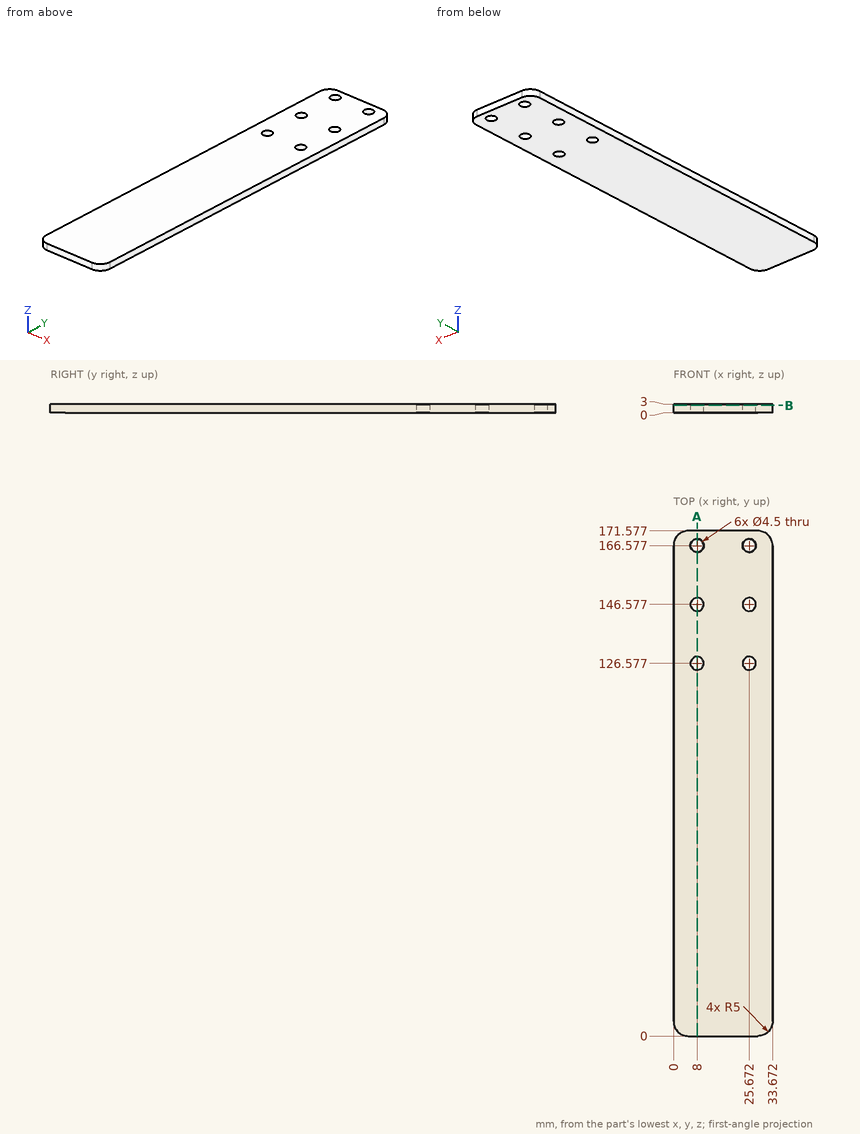
Check sheet for the drawn part. Datum: minimum x, y, z corner. Units: mm. Round coordinates to 2 decimals unless told otherwise and drop trailing zeros. Loops run counter-clockwise (first coordinate to the right, second up) from the corner with the lowest first, then second, coordinate; pieces in that order, holes last.
Item 1: Cross-section at A-A on x = 8. Record the boundary of the cut face in (y, z).
Item 2: Cross-section at B-B on z = 2.5. Record the boundary of the cut face in (x, y), then the cut area to 3 significant figures.
Item 3: Thickness scan on line 1 (Y direction, x = 8, z = 1.05); line 2 (X direction, y = 147.5, z = 0.65); line 3 (Y direction, x = 25, z = 2.35) (1 decimal). Record the ranges inside material, lowest first.
Answer sheet:
1. outline: (0, 0) - (124.33, 0) - (124.33, 3) - (0, 3) - close; (128.83, 0) - (144.33, 0) - (144.33, 3) - (128.83, 3) - close; (148.83, 0) - (164.33, 0) - (164.33, 3) - (148.83, 3) - close; (168.83, 0) - (171.58, 0) - (171.58, 3) - (168.83, 3) - close
2. outline: (0, 5) arc R5 ccw to (5, 0) - (28.67, 0) arc R5 ccw to (33.67, 5) - (33.67, 166.58) arc R5 ccw to (28.67, 171.58) - (5, 171.58) arc R5 ccw to (0, 166.58) - close; hole circle Ø4.5 at (8, 126.58); hole circle Ø4.5 at (8, 146.58); hole circle Ø4.5 at (8, 166.58); hole circle Ø4.5 at (25.67, 126.58); hole circle Ø4.5 at (25.67, 146.58); hole circle Ø4.5 at (25.67, 166.58)
2. area: 5,660 mm2
3. line 1: y = 0 to 124.33, 128.83 to 144.33, 148.83 to 164.33, 168.83 to 171.58
3. line 2: x = 0 to 5.95, 10.05 to 23.62, 27.72 to 33.67
3. line 3: y = 0 to 124.4, 128.7 to 144.4, 148.7 to 164.4, 168.7 to 171.6
